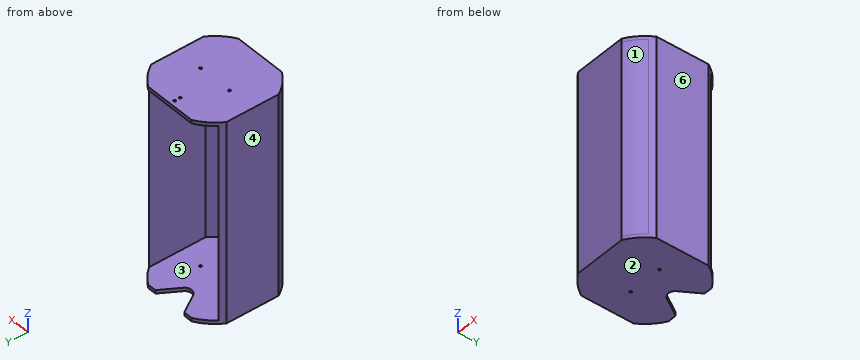
Autodesk Inventor part; units mm, degrees
ref_plane "YZ Plane" through (0, 0, 0) normal (1, 0, 0) x (0, 1, 0)
ref_plane "XZ Plane" through (0, 0, 0) normal (0, 1, 0) x (-1, 0, 0)
ref_plane "XY Plane" through (0, 0, 0) normal (0, 0, 1) x (1, 0, 0)
sketch "Sketch1" plane through (0, 0, 0) normal (0, 1, 0) x (-1, 0, 0)
  line L0 (-65, 145) -> (65, 145)
  line L1 (65, 145) -> (65, -145)
  line L2 (65, -145) -> (-65, -145)
  line L3 (-65, -145) -> (-65, 145)
  line L4 (-65, 145) -> (65, -145) construction
  line L5 (65, 145) -> (-65, -145) construction
  point P0 (0, 0)
  dimension "d0" = 130
  dimension "d1" = 290
extrude "Extrusion1" add sketch "Sketch1" along normal blind 130
sketch "Sketch2" plane through (-65, 0, 145) normal (0, 0, 1) x (1, 0, 0)
  line L0 (0, 0) -> (130, 0)
  line L1 (130, 0) -> (130, 130)
  line L2 (0, 130) -> (130, 130)
  line L3 (0, 0) -> (0, 130)
  circle A0 centre (65, 65) radius 75
  point P0 (65, 0)
  point P1 (130, 65)
  point P2 (65, 130)
  point P3 (27.5834, 0)
  point P4 (0, 27.5834)
  point P5 (130, 27.5834)
  point P6 (102.4166, 0)
  point P7 (0, 102.4166)
  point P8 (27.5834, 130)
  point P9 (102.4166, 130)
  point P10 (130, 102.4166)
  dimension "d4" = 150
extrude "Extrusion2" cut sketch "Sketch2" against normal through all contours L3 A0 L0 | A0 L1 L0 | L3 L2 A0 | A0 L2 L1
sketch "Sketch3" plane through (0, 130, 0) normal (0, 1, 0) x (1, 0, 0)
  line L0 (-37.4166, 145) -> (-37.4166, -145)
  line L1 (-37.4166, -145) -> (37.4166, -145)
  line L2 (37.4166, -145) -> (37.4166, 145)
  line L3 (37.4166, 145) -> (-37.4166, 145)
  line L4 (37.4166, 145) -> (65, 145)
  line L5 (37.4166, -145) -> (37.4166, 145)
  line L6 (65, -145) -> (37.4166, -145)
  line L7 (65, 145) -> (65, -145)
  line L8 (-65, 145) -> (-37.4166, 145)
  line L9 (-65, -145) -> (-65, 145)
  line L10 (-37.4166, -145) -> (-65, -145)
  line L11 (-37.4166, 145) -> (-37.4166, -145)
  line L12 (-60, -140) -> (60, -140)
  line L13 (60, -140) -> (60, 140)
  line L14 (60, 140) -> (-60, 140)
  line L15 (-60, 140) -> (-60, -140)
  line L16 (-60, -140) -> (60, 140) construction
  line L17 (60, -140) -> (-60, 140) construction
  point P0 (0, 0)
  dimension "d7" = 5
  dimension "d8" = 5
extrude "Extrusion3" cut sketch "Sketch3" against normal through all contours L14 L2 L12 L0 | L0 L12 L15 L14 | L14 L13 L12 L2
sketch "Sketch4" plane through (-37.4166, 0, 145) normal (0, 0, 1) x (1, 0, 0)
  arc A0 (74.8331, 0) -> (102.4166, 27.5834) centre (37.4166, 65) ccw
  line L0 (102.4166, 27.5834) -> (102.4166, 102.4166)
  arc A1 (102.4166, 102.4166) -> (74.8331, 130) centre (37.4166, 65) ccw
  line L1 (0, 130) -> (74.8331, 130)
  arc A2 (0, 130) -> (-27.5834, 102.4166) centre (37.4166, 65) ccw
  line L2 (-27.5834, 27.5834) -> (-27.5834, 102.4166)
  arc A3 (-27.5834, 27.5834) -> (0, 0) centre (37.4166, 65) ccw
  line L3 (0, 0) -> (74.8331, 0)
  arc A4 (-22.5834, 28.9445) -> (1.3611, 5) centre (37.4166, 65) ccw
  line L4 (-22.5834, 28.9445) -> (-22.5834, 101.0555)
  arc A5 (1.3611, 125) -> (-22.5834, 101.0555) centre (37.4166, 65) ccw
  line L5 (1.3611, 125) -> (73.4721, 125)
  arc A6 (97.4166, 101.0555) -> (73.4721, 125) centre (37.4166, 65) ccw
  line L6 (97.4166, 101.0555) -> (97.4166, 28.9445)
  arc A7 (73.4721, 5) -> (97.4166, 28.9445) centre (37.4166, 65) ccw
  line L7 (73.4721, 5) -> (1.3611, 5)
  line L8 (-27.5834, 27.5834) -> (-22.5834, 28.9445)
  line L9 (97.4166, 28.9445) -> (102.4166, 27.5834)
  point P0 (37.4166, 0)
  dimension "d11" = 5
extrude "Extrusion4" add sketch "Sketch4" against normal up to surface (290 mm away) contours L3 A3 L8 A4 L7 A7 L9 A0
sketch "Sketch5" plane through (-37.4166, 0, 145) normal (0, 0, 1) x (1, 0, 0)
  line L0 (102.4166, 27.5834) -> (102.4166, 102.4166)
  arc A0 (102.4166, 102.4166) -> (74.8331, 130) centre (37.4166, 65) ccw
  line L1 (0, 130) -> (74.8331, 130)
  arc A1 (0, 130) -> (-27.5834, 102.4166) centre (37.4166, 65) ccw
  line L2 (-27.5834, 27.5834) -> (-27.5834, 102.4166)
  arc A2 (-27.5834, 27.5834) -> (0, 0) centre (37.4166, 65) ccw
  line L3 (0, 0) -> (74.8331, 0)
  arc A3 (74.8331, 0) -> (102.4166, 27.5834) centre (37.4166, 65) ccw
  line L4 (12.4166, 65) -> (62.4166, 65) construction
  circle A4 centre (62.4166, 65) radius 1.65
  circle A5 centre (12.4166, 65) radius 1.65
  point P0 (37.4166, 0)
  dimension "d14" = 3.3
  dimension "d15" = 3.3
  dimension "d16" = 50
extrude "Extrusion5" cut sketch "Sketch5" against normal through all contours A4 | A5
sketch "Sketch7" plane through (37.4166, 0, -145) normal (0, 0, -1) x (-1, 0, 0)
  circle A0 centre (12.4166, 65) radius 1.65
  circle A1 centre (62.4166, 65) radius 1.65
  arc A2 (-27.5834, 27.5834) -> (0, 0) centre (37.4166, 65) ccw
  line L0 (0, 0) -> (74.8331, 0)
  arc A3 (74.8331, 0) -> (102.4166, 27.5834) centre (37.4166, 65) ccw
  line L1 (102.4166, 27.5834) -> (102.4166, 102.4166)
  arc A4 (102.4166, 102.4166) -> (74.8331, 130) centre (37.4166, 65) ccw
  line L2 (0, 130) -> (74.8331, 130)
  arc A5 (0, 130) -> (-27.5834, 102.4166) centre (37.4166, 65) ccw
  line L3 (-27.5834, 27.5834) -> (-27.5834, 102.4166)
  line L4 (12.4166, 130) -> (28.9366, 103.568)
  line L5 (45.8966, 103.568) -> (62.4166, 130)
  arc A6 (28.9366, 103.568) -> (45.8966, 103.568) centre (37.4166, 108.868) ccw
  point P0 (37.4166, 0)
  point P1 (37.4166, 90)
  dimension "d24" = 50
  dimension "d25" = 40
  dimension "d26" = 10
extrude "Extrusion7" cut sketch "Sketch7" against normal blind 10 contours L2 L5 A6 L4
sketch "Sketch10" plane through (37.4166, 130, 140) normal (0, 0, -1) x (-1, 0, 0)
  circle A0 centre (12.4166, -65) radius 1.65
  circle A1 centre (62.4166, -65) radius 1.65
  arc A2 (73.4721, -125) -> (97.4166, -101.0555) centre (37.4166, -65) ccw
  line L0 (97.4166, -20) -> (97.4166, -101.0555)
  arc A3 (97.4166, -20) -> (74.8331, 0) centre (37.4166, -65) ccw
  line L1 (0, 0) -> (74.8331, 0)
  arc A4 (0, 0) -> (-22.5834, -20) centre (37.4166, -65) ccw
  line L2 (-22.5834, -20) -> (-22.5834, -101.0555)
  arc A5 (-22.5834, -101.0555) -> (1.3611, -125) centre (37.4166, -65) ccw
  line L3 (1.3611, -125) -> (73.4721, -125)
  circle A6 centre (37.4166, -7) radius 1.65
  circle A7 centre (37.4166, -15) radius 1.65
  point P0 (37.4166, -130)
  point P1 (37.4166, 0)
  dimension "d36" = 3.3
  dimension "d37" = 3.3
  dimension "d38" = 8
  dimension "d39" = 7
extrude "Extrusion10" cut sketch "Sketch10" against normal through all contours A6 | A7
sketch "Sketch11" plane through (37.4166, 130, 140) normal (0, 0, -1) x (-1, 0, 0)
  circle A0 centre (37.4166, -15) radius 1.65
  circle A1 centre (37.4166, -7) radius 1.65
  circle A2 centre (12.4166, -65) radius 1.65
  circle A3 centre (62.4166, -65) radius 1.65
  arc A4 (73.4721, -125) -> (97.4166, -101.0555) centre (37.4166, -65) ccw
  line L0 (97.4166, -20) -> (97.4166, -101.0555)
  arc A5 (97.4166, -20) -> (74.8331, 0) centre (37.4166, -65) ccw
  line L1 (0, 0) -> (74.8331, 0)
  arc A6 (0, 0) -> (-22.5834, -20) centre (37.4166, -65) ccw
  line L2 (-22.5834, -20) -> (-22.5834, -101.0555)
  arc A7 (-22.5834, -101.0555) -> (1.3611, -125) centre (37.4166, -65) ccw
  line L3 (1.3611, -125) -> (73.4721, -125)
  circle A8 centre (37.4166, -7) radius 2.9
  circle A9 centre (37.4166, -15) radius 2.9
  point P0 (37.4166, -130)
  dimension "d42" = 5.8
extrude "Extrusion11" cut sketch "Sketch11" against normal blind 3 contours A0 | A1 | A8 | A9
properties part number "CAJA_V2" material "Steel, Mild, Welded"
For this review, take the finished solid that the model builds, in its own axes (mm). Face numbers are marked on the shaded views. A direction names the side the tool comes from. Round coordinates to 2 decimals unless told otherwise and drop trailing zeros. Loops run counter-clockwise (first coordinate to the right, second up) from the corner with the lowest first, then second, coordinate; pieces in that order, holes last.
(1) We need section D-D (y = 13.5). Give the boundary of the cut face in (x, z).
Returned:
outline: (-54.52, -145) - (54.52, -145) - (54.52, 145) - (-54.52, 145) - close; hole (-47.41, -140) - (47.41, -140) - (47.41, 140) - (-47.41, 140) - close
(2) Tool access review of the marked faces 5 and 6: name each direction out of +Z, -Z, +X, -X, +Y, -Y from which nothing blocks a thin tool from reaching the whole face with its end or side.
Returned:
face 5: +Y
face 6: +Z, -Z, +X, +Y, -Y
(3) We need section C-C (z = -29). Give the boundary of the cut face in (x, y), plus the area to 3 significant figures.
Returned:
outline: (-65, 27.58) arc R75 ccw to (-37.42, 0) - (37.42, 0) arc R75 ccw to (60, 20) arc R75 ccw to (65, 27.58) - (65, 102.42) arc R75 ccw to (60, 110) - (60, 28.94) arc R70 cw to (36.06, 5) - (-36.06, 5) arc R70 cw to (-60, 28.94) - (-60, 110) arc R75 ccw to (-65, 102.42) - close
area: 1,520 mm2
(4) Wall thickness on line 1 along X through (y, z) = (65, 143); line 2 along Y through (x, z) = (0, 143.65); line 3 along Y through (x, z) = (0, 141.6): over which ranges is each line inside the solid? List them lowest first.
Returned:
line 1: x = -65 to -26.65, -23.35 to 23.35, 26.65 to 65
line 2: y = 0 to 113.35, 116.65 to 121.35, 124.65 to 130
line 3: y = 0 to 112.1, 117.9 to 120.1, 125.9 to 130
(5) Clearance check with flat-ended pins moving along their axes: P1, Ø4.5, axis at x = 0, y = 114, coming from the -Z side; P2, Ø10, axis at y = 113.5, z = -38.5, coming from the +X side; P3, Ø5.5, axis at x = 0, y = 123, coming from the -Z side. State where each tip first meets the part, or that it passes through.
Returned:
P1: stops at z = 140
P2: stops at x = 61.1
P3: stops at z = 143
(6) We need section B-B (y = 58.5). Give the boundary of the cut face in (x, z).
Returned:
outline: (-65, -145) - (65, -145) - (65, 145) - (-65, 145) - close; hole (-60, -140) - (60, -140) - (60, 140) - (-60, 140) - close
(7) Mouldability with a two-part tool opening along X and no side actions: class the marked faces 1, 2, 3 and 4 as released by +X, released by -X, zero draft, split by the parting line, or undercut.
Returned:
face 1: released by +X
face 2: zero draft
face 3: undercut
face 4: released by -X
(8) We need section A-A (x = 20.5). Give the boundary of the cut face in (y, z).
Returned:
outline: (0, -145) - (122.8, -145) - (122.8, -140) - (5, -140) - (5, 140) - (130, 140) - (130, 145) - (0, 145) - close
